Part model, mm, in its own coordinate system. A direction names the side the tool comes from. Coordinates: 2 decimals unless noted, no trailing zeros. Order: outer loops, then holes, each group sorted by start corner. A loop starts at its lowest first (then second) coordinate and runs counter-clockwise, first axis right, second up.
Autodesk Inventor part; units mm, degrees
ref_plane "YZ Plane" through (0, 0, 0) normal (1, 0, 0) x (0, 1, 0)
ref_plane "XZ Plane" through (0, 0, 0) normal (0, 1, 0) x (-1, 0, 0)
ref_plane "XY Plane" through (0, 0, 0) normal (0, 0, 1) x (1, 0, 0)
sketch "Skizze1" plane through (0, 0, 0) normal (0, 1, 0) x (-1, 0, 0)
  line L0 (0, 50) -> (13.5, 50)
  line L1 (13.5, 50) -> (13.5, 41)
  line L2 (13.5, 41) -> (14.6, 41)
  line L3 (14.6, 41) -> (14.6, 0)
  line L4 (14.6, 0) -> (0, 0)
  line L5 (0, 0) -> (0, 50)
  line L6 (14.6, 26) -> (13.6, 26)
  line L7 (13.6, 26) -> (13.6, 25.5)
  line L8 (13.6, 25.5) -> (14.6, 25.5)
  line L9 (14.6, 25.5) -> (14.6, 26)
  line L10 (0, 0) -> (13.95, 0)
  line L11 (13.95, 0) -> (13.95, -2.7)
  line L12 (13.95, -2.7) -> (0, -2.7)
  line L13 (0, -2.7) -> (0, 0)
  line L14 (0, -2.7) -> (12.5, -2.7)
  line L15 (12.5, -2.7) -> (12.5, -7.7)
  line L16 (12.5, -7.7) -> (0, -7.7)
  line L17 (0, -7.7) -> (0, -2.7)
  point P0 (14.1, 25.5)
  point P1 (13.6, 25.75)
  point P2 (14.1, 26)
  point P3 (14.05, 41)
  point P4 (13.95, 0)
  dimension "d0" = 13.5
  dimension "d1" = 9
  dimension "d2" = 90
  dimension "d3" = 1.1
  dimension "d4" = 270
  dimension "d5" = 0.5
  dimension "d6" = 1
  dimension "d7" = 15
  dimension "d9" = 13.95
  dimension "d10" = 2.7
  dimension "d13" = 12.5
  dimension "d14" = 5
revolve "Umdrehung1" add sketch "Skizze1" angle 360 about axis through (0, 0, 0) along (0, 0, 1) contours L0 L1 L2 L3 L6 L7 L8 L4 L5 | L4 L11 L12 L13 | L12 L15 L16 L17
thread "Gewinde1"
properties part number "00_CCTV_Lens_Hikvision_50mm_2.8"
(1) Probe line 1 (Y direction, x = 0.5, z = -4.5); line 2 (Y direction, x = -0.5, z = 44); line 3 (X direction, y = 1.5, z = 33). List the from-to ranges inside material, lowest first.
(2) Drop flat-ended pins along their axis: pin 1 (2 mm diameter, centred on x = -9, z = 13.5, fed in from +Y); pin 2 (3 mm diameter, centred on y = -5, z = 18.5, fed in from -X); pin 3 (5 mm diameter, centred on x = -8.5, z = 25.5, fed in from -Y). Give the stop position or say it passes through.
(3) Tool access for faces 1 (the face through (-13.926, 4.385, 12.572)), 2 (the face through (2.93, -13.18, 45.44)), 3 (the face through (12, -7, 25.5)), 4 (the face through (-11.923, 3.755, -5.235)): list every direction of +Z, -Z, +X, -X, +Y, -Y with a clear straight run to the whole face (end or side of a thin tool).
(4) Slice it at C-C, the plane z = 15. Give the cut face in (x, y).
(5) Pull direction Z, two halves, no side cores. Call faces 5 (the face through (0, 0, -7.7)), 6 (the face through (-10, 10, 41)), 7 (the face through (12, -7, 26)), 8 (the face through (2.948, -13.277, 25.746)): +Z half, -Z half, draft (parallel to the pull), parting line (faces both ways), or undercut.
(6) Slice it at A-A, the plane x = 0. Give the cut face in (y, z).
Here are the results:
1. line 1: y = -12.49 to 12.49
1. line 2: y = -13.49 to 13.49
1. line 3: x = -14.52 to 14.52
2. pin 1: stops at y = 12.21
2. pin 2: stops at x = -14.17
2. pin 3: stops at y = -13.31
3. face 1: +Z, -Z
3. face 2: +Z
3. face 3: none
3. face 4: -Z
4. outline: circle Ø29.2 at (0, 0)
5. face 5: -Z half
5. face 6: +Z half
5. face 7: undercut
5. face 8: undercut
6. outline: (-14.6, 0) - (-13.95, 0) - (-13.95, -2.7) - (-12.5, -2.7) - (-12.5, -7.7) - (12.5, -7.7) - (12.5, -2.7) - (13.95, -2.7) - (13.95, 0) - (14.6, 0) - (14.6, 25.5) - (13.6, 25.5) - (13.6, 26) - (14.6, 26) - (14.6, 41) - (13.5, 41) - (13.5, 50) - (-13.5, 50) - (-13.5, 41) - (-14.6, 41) - (-14.6, 26) - (-13.6, 26) - (-13.6, 25.5) - (-14.6, 25.5) - close
